```python
from build123d import *

# Parameters (mm, degrees)
F0_W     = 70
F0_H     = 70
F1_DEPTH = 2.5
F2_W     = 10
F2_H     = 5
F3_DEPTH = 5
F4_W     = 5
F4_H     = 10
F5_DEPTH = 5
F7_D     = 6.6


with BuildPart() as f1:
    # F0 (on Right) → F1 (new body, symmetric)
    with BuildSketch(Plane.YZ):
        Rectangle(F0_W, F0_H)
    extrude(amount=F1_DEPTH, both=True)

    # F2 (on face) → F3 (join)
    with BuildSketch(Plane.YZ.offset(2.5)):
        with Locations((-20, -37.5)):
            Rectangle(F2_W, F2_H)
        with Locations((0, -37.5)):
            Rectangle(F2_W, F2_H)
        with Locations((20, -37.5)):
            Rectangle(F2_W, F2_H)
    extrude(amount=-F3_DEPTH)

    # F4 (on face) → F5 (join, through all)
    with BuildSketch(Plane.YZ.offset(2.5)):
        with Locations((-37.5, -30)):
            Rectangle(F4_W, F4_H)
        with Locations((-37.5, -10)):
            Rectangle(F4_W, F4_H)
        with Locations((-37.5, 10)):
            Rectangle(F4_W, F4_H)
        with Locations((-37.5, 30)):
            Rectangle(F4_W, F4_H)
        with Locations((37.5, 30)):
            Rectangle(F4_W, F4_H)
        with Locations((37.5, -30)):
            Rectangle(F4_W, F4_H)
        with Locations((37.5, 10)):
            Rectangle(F4_W, F4_H)
        with Locations((37.5, -10)):
            Rectangle(F4_W, F4_H)
    extrude(amount=-F5_DEPTH)

    # F7 (through all)
    with Locations(Plane.YZ.offset(2.5)):
        with Locations((-17.6776695297, 21.6776695297), (17.6776695297, 21.6776695297), (17.6776695297, -13.6776695297), (-17.6776695297, -13.6776695297)):
            Hole(F7_D / 2)


solid = f1.part
```
The model under review builds one solid part; all positions refer to its coordinate system, in mm. A direction names the side the tool comes from. Round coordinates to 2 decimals unless told otherwise and drop trailing zeros. Order: outer loops, then holes, each group sorted by start corner. A loop starts at its lowest first (then second) coordinate and runs counter-clockwise, first axis right, second up. Notation, with made-up numbers: (52.25, 9) -> (96.25, 9) arc R16 cw to (96.25, 38) -> close; hole circle Ø5 at (50, 70). An arc over 180 degrees is marked (long way). One line per item, written item: value. Start each with the question number.
Q1. Take a section at A-A (y = -18). Write out the cut boundary in (x, z).
Q2. Machinability: for faces 1 (the face through (0, 10, -35)), 2 (the face through (0, -33, -35)), 3 (the face through (0, -38, 15)), 4 (the face through (0, 37, 15)), 5 (the face through (0, 32, -35)), which of the approach directions +Z, -Z, +X, -X, +Y, -Y give a long, thin tool a straight path to every point of the face, cutting with its end or side? Answer none if there is none.
Q3. Clearance check with flat-ended pins moving along their axes: pin 1 Ø6 at (y, z) = (17.68, 21.68) entering from -X; pin 2 Ø1.5 at (x, y) = (-1, -10) entering from -Z; pin 3 Ø8.5 at (y, z) = (17.68, -13.68) entering from +X; pin 4 Ø1.5 at (x, z) = (-1, 18.5) entering from +Y. State where each tip first meets the part, or that it passes through.
Q4. Take a section at B-B (z = 16.5). Write out the cut boundary in (x, y).
Q5. Mouldability with a two-part tool opening along Z and no side actions: class faces 6 (the face through (0, 0, -40)), 7 (the face through (0, 5, -38)), 8 (the face through (0, -38, -15)), 9 (the face through (0, -38, -5)) as released by +Z, released by -Z, zero draft, split by the parting line, or undercut.
Q6. Wall thickness on line 1 (Z direction, x = -2.15, y = -36); line 2 (Y direction, x = -0.8, z = -35.5); line 3 (Z direction, x = 1.95, y = -18.5): over which ranges is each line inside the solid? List them lowest first.
Q7. Take a section at C-C (x = -0.8). Count the separate pieces of the cut face and the enclosed holes in it, and give its area (3 significant figures).
Reported:
1. outline: (-2.5, -40) -> (2.5, -40) -> (2.5, -16.96) -> (-2.5, -16.96) -> close; (-2.5, -10.39) -> (2.5, -10.39) -> (2.5, 18.39) -> (-2.5, 18.39) -> close; (-2.5, 24.96) -> (2.5, 24.96) -> (2.5, 35) -> (-2.5, 35) -> close
2. face 1: -Z, +X, -X
2. face 2: -Z, +X, -X, -Y
2. face 3: +X, -X, -Y
2. face 4: +X, -X, +Y
2. face 5: -Z, +X, -X, +Y
3. pin 1: passes through
3. pin 2: stops at z = -35
3. pin 3: stops at x = 2.5
3. pin 4: stops at y = 35
4. outline: (-2.5, -35) -> (2.5, -35) -> (2.5, 35) -> (-2.5, 35) -> close
5. face 6: released by -Z
5. face 7: zero draft
5. face 8: undercut
5. face 9: undercut
6. line 1: z = -35 to -25, -15 to -5, 5 to 15, 25 to 35
6. line 2: y = -25 to -15, -5 to 5, 15 to 25
6. line 3: z = -40 to -16.87, -10.48 to 18.48, 24.87 to 35
7. separate pieces: 1
7. enclosed holes: 4
7. area: 5,310 mm2
